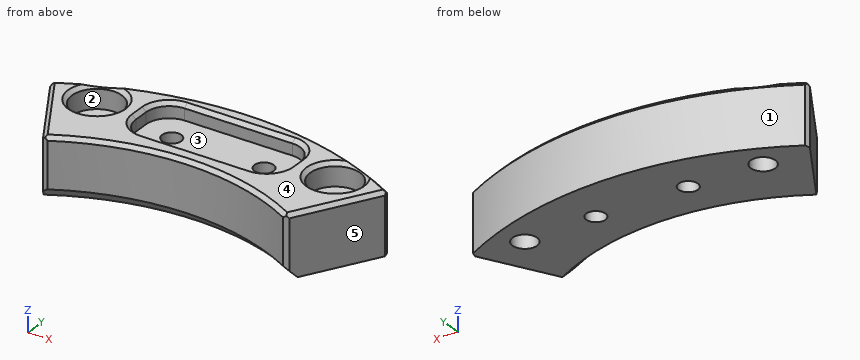
from build123d import *

# Parameters (mm, degrees)
EXTRUDE_1_DEPTH              = 8
CHAMFER_7_SIZE               = 1.5
HOLE_WIZARD_M3_1_D           = 3.2
HOLE_WIZARD_M3_1_CBORE_D     = 6.5
HOLE_WIZARD_M3_1_CBORE_DEPTH = 3
CUT_EXTRUDE_6_DEPTH          = 2
CHAMFER_8_SIZE               = 0.5
CHAMFER_9_SIZE               = 0.5
M3X0_5_1_D                   = 2.5
M3X0_5_1_DEPTH               = 8.5
M3X0_5_1_TIP                 = 0.751075774


with BuildPart() as part:
    # ｽｹｯﾁ3 → ﾎﾞｽ - 押し出し1 (new body)
    with BuildSketch(Plane.XY.offset(-16.5)):
        with BuildLine():
            Line((58.49999999, 38.105482977), (64.74999999, 27.280165429))
            ThreePointArc((64.74999999, 27.280165429), (80.49999999, 31.50036521), (96.24999999, 27.280165429))
            Line((96.24999999, 27.280165429), (102.49999999, 38.105482977))
            ThreePointArc((102.49999999, 38.105482977), (80.49999999, 44.00036521), (58.49999999, 38.105482977))
        make_face()
    extrude(amount=EXTRUDE_1_DEPTH)

    # 面取り7
    chamfer_7_edges = [part.edges().sort_by_distance(p)[0] for p in [
        (80.49999999, 31.50036521, -16.5),
    ]]
    chamfer(chamfer_7_edges, length=CHAMFER_7_SIZE)

    # M3 穴付きねじ用座ぐり穴1 (through all)
    with Locations(Plane.XY.offset(-8.5)):
        with Locations((65.0229264, 37.390950693), (95.977073581, 37.390950693)):
            CounterBoreHole(HOLE_WIZARD_M3_1_D / 2, HOLE_WIZARD_M3_1_CBORE_D / 2, HOLE_WIZARD_M3_1_CBORE_DEPTH)

    # ｽｹｯﾁ17 → ｶｯﾄ - 押し出し6 (cut)
    with BuildSketch(Plane.XY.offset(-8.5)):
        with BuildLine():
            Line((73.49999999, 41.75036521), (87.49999999, 41.75036521))
            ThreePointArc((87.49999999, 41.75036521), (89.621320334, 40.871685554), (90.49999999, 38.75036521))
            Line((90.49999999, 38.75036521), (90.49999999, 36.75036521))
            ThreePointArc((90.49999999, 36.75036521), (89.621320334, 34.629044867), (87.49999999, 33.75036521))
            Line((87.49999999, 33.75036521), (73.49999999, 33.75036521))
            ThreePointArc((73.49999999, 33.75036521), (71.378679647, 34.629044867), (70.49999999, 36.75036521))
            Line((70.49999999, 36.75036521), (70.49999999, 38.75036521))
            ThreePointArc((70.49999999, 38.75036521), (71.378679647, 40.871685554), (73.49999999, 41.75036521))
        make_face()
    extrude(amount=-CUT_EXTRUDE_6_DEPTH, mode=Mode.SUBTRACT)

    # 面取り8
    # the kernel refuses this chamfer: 0.5 mm, written as the material it takes off along each edge
    with BuildSketch(Plane(origin=(80.49999999, 0.00036521, -8.5), x_dir=(-0.5349312949950591, 0.844895561377209, 0), z_dir=(-0.844895561377209, -0.5349312949950591, 0))) as chamfer_8_piece_1:
        Polygon((31.5, CHAMFER_8_SIZE), (31.5 + CHAMFER_8_SIZE, 0), (31.5, 0), align=None)
    revolve(axis=Axis((80.49999999, 0.00036521, -8.5), (0, 0, -1)), revolution_arc=64.678504259, mode=Mode.SUBTRACT)
    with BuildSketch(Plane(origin=(95.607079243, 26.16659403, -8.5), x_dir=(-0.8660254037844379, 0.5000000000000012, 0), z_dir=(0.5000000000000012, 0.866025403784438, 0))) as chamfer_8_piece_2:
        Polygon((CHAMFER_8_SIZE, 0), (0, -CHAMFER_8_SIZE), (0, 0), align=None)
    extrude(amount=15.071682988, mode=Mode.SUBTRACT)
    with BuildSketch(Plane(origin=(80.49999999, 0.00036521, -8.5), x_dir=(0.5250957878127545, 0.8510431326444641, 0), z_dir=(0.8510431326444641, -0.5250957878127545, 0))) as chamfer_8_piece_3:
        Polygon((44 - CHAMFER_8_SIZE, 0), (44, -CHAMFER_8_SIZE), (44, 0), align=None)
    revolve(axis=Axis((80.49999999, 0.00036521, -8.5), (0, 0, 1)), revolution_arc=63.349383731, mode=Mode.SUBTRACT)
    with BuildSketch(Plane(origin=(95.977073581, 37.390950693, -8.5), x_dir=(1, 0, 0), z_dir=(0, -1, 0))) as chamfer_8_piece_4:
        Polygon((3.25 + CHAMFER_8_SIZE, 0), (3.25, -CHAMFER_8_SIZE), (3.25, 0), align=None)
    revolve(axis=Axis((95.977073581, 37.390950693, -8.5), (0, 0, 1)), mode=Mode.SUBTRACT)
    with BuildSketch(Plane(origin=(65.0229264, 37.390950693, -8.5), x_dir=(1, 0, 0), z_dir=(0, -1, 0))) as chamfer_8_piece_5:
        Polygon((3.25 + CHAMFER_8_SIZE, 0), (3.25, -CHAMFER_8_SIZE), (3.25, 0), align=None)
    revolve(axis=Axis((65.0229264, 37.390950693, -8.5), (0, 0, 1)), mode=Mode.SUBTRACT)
    with BuildSketch(Plane(origin=(57.857079243, 39.219054376, -8.5), x_dir=(0, 0, -1), z_dir=(0.5000000000000007, -0.8660254037844384, 0))) as chamfer_8_piece_6:
        Polygon((CHAMFER_8_SIZE, 0), (0, CHAMFER_8_SIZE), (0, 0), align=None)
    extrude(amount=15.071682988, mode=Mode.SUBTRACT)
    with BuildSketch(Plane(origin=(87.49999999, 38.75036521, -8.5), x_dir=(0, 1, 0), z_dir=(-1, 0, 0))) as chamfer_8_piece_7:
        Polygon((3 + CHAMFER_8_SIZE, 0), (3, CHAMFER_8_SIZE), (3, 0), align=None)
    revolve(axis=Axis((87.49999999, 38.75036521, -8.5), (0, 0, -1)), revolution_arc=90, mode=Mode.SUBTRACT)
    with BuildSketch(Plane(origin=(73.49999999, 41.75036521, -8.5), x_dir=(0, 1, 0), z_dir=(1, 0, 0)), Plane(origin=(87.49999999, 33.75036521, -8.5), x_dir=(0, -1, 0), z_dir=(-1, 0, 0))) as chamfer_8_piece_8:
        Polygon((CHAMFER_8_SIZE, 0), (0, -CHAMFER_8_SIZE), (0, 0), align=None)
    extrude(amount=14, mode=Mode.SUBTRACT)
    with BuildSketch(Plane(origin=(73.49999999, 38.75036521, -8.5), x_dir=(-1, 0, 0), z_dir=(0, -1, 0))) as chamfer_8_piece_9:
        Polygon((3 + CHAMFER_8_SIZE, 0), (3, CHAMFER_8_SIZE), (3, 0), align=None)
    revolve(axis=Axis((73.49999999, 38.75036521, -8.5), (0, 0, -1)), revolution_arc=90, mode=Mode.SUBTRACT)
    with BuildSketch(Plane(origin=(70.49999999, 36.75036521, -8.5), x_dir=(-1, 0, 0), z_dir=(0, 1, 0)), Plane(origin=(90.49999999, 38.75036521, -8.5), x_dir=(1, 0, 0), z_dir=(0, -1, 0))) as chamfer_8_piece_10:
        Polygon((CHAMFER_8_SIZE, 0), (0, -CHAMFER_8_SIZE), (0, 0), align=None)
    extrude(amount=2, mode=Mode.SUBTRACT)
    with BuildSketch(Plane(origin=(73.49999999, 36.75036521, -8.5), x_dir=(0, -1, 0), z_dir=(1, 0, 0))) as chamfer_8_piece_11:
        Polygon((3 + CHAMFER_8_SIZE, 0), (3, CHAMFER_8_SIZE), (3, 0), align=None)
    revolve(axis=Axis((73.49999999, 36.75036521, -8.5), (0, 0, -1)), revolution_arc=90, mode=Mode.SUBTRACT)
    with BuildSketch(Plane(origin=(87.49999999, 36.75036521, -8.5), x_dir=(1, 0, 0), z_dir=(0, 1, 0))) as chamfer_8_piece_12:
        Polygon((3 + CHAMFER_8_SIZE, 0), (3, CHAMFER_8_SIZE), (3, 0), align=None)
    revolve(axis=Axis((87.49999999, 36.75036521, -8.5), (0, 0, -1)), revolution_arc=90, mode=Mode.SUBTRACT)

    # 面取り9
    # the kernel refuses this chamfer: 0.5 mm, written as the material it takes off along each edge
    with BuildSketch(Plane(origin=(96.24999999, 27.280165429, -16.296233904), x_dir=(-0.8699980733677616, 0.4930551209919465, 0), z_dir=(0, 0, 1))) as chamfer_9_piece_1:
        with BuildLine():
            Line((0.504048916, 0), (-CHAMFER_9_SIZE * 0.00800077643885, -CHAMFER_9_SIZE * 0.999967993276))
            Line((-CHAMFER_9_SIZE * 0.00800077643885, -CHAMFER_9_SIZE * 0.999967993276), (0, 0))
            ThreePointArc((0, 0), (0.259153689, -0.001007405), (0.504048916, 0))
        make_face()
    extrude(amount=8.592467809, mode=Mode.SUBTRACT)
    with BuildSketch(Plane(origin=(64.74999999, 27.280165429, -16.296233904), x_dir=(-0.499999999999999, 0.8660254037844393, 0), z_dir=(0, 0, 1))) as chamfer_9_piece_2:
        with BuildLine():
            Line((CHAMFER_9_SIZE, 0), (-0.004032783, -0.504032783))
            ThreePointArc((-0.004032783, -0.504032783), (-0.001066058, -0.259153454), (0, 0))
            Line((0, 0), (CHAMFER_9_SIZE, 0))
        make_face()
    extrude(amount=8.592467809, mode=Mode.SUBTRACT)
    with BuildSketch(Plane(origin=(58.49999999, 38.105482977, -17.785841494), x_dir=(0.5000000000000021, -0.8660254037844375, 0), z_dir=(0, 0, 1))) as chamfer_9_piece_3:
        with BuildLine():
            Line((CHAMFER_9_SIZE, 0), (0.002809166, 0.497190834))
            ThreePointArc((0.002809166, 0.497190834), (0.000742578, 0.255629249), (0, 0))
            Line((0, 0), (CHAMFER_9_SIZE, 0))
        make_face()
    extrude(amount=10.071682988, mode=Mode.SUBTRACT)
    with BuildSketch(Plane(origin=(102.49999999, 38.105482977, -17.785841494), x_dir=(-0.8688365739050292, 0.4950989879256175, 0), z_dir=(0, 0, 1))) as chamfer_9_piece_4:
        with BuildLine():
            Line((0.49719877, 0), (CHAMFER_9_SIZE * 0.00564998602096, CHAMFER_9_SIZE * 0.999984038702))
            Line((CHAMFER_9_SIZE * 0.00564998602096, CHAMFER_9_SIZE * 0.999984038702), (0, 0))
            ThreePointArc((0, 0), (0.255629364, -0.000701736), (0.49719877, 0))
        make_face()
    extrude(amount=10.071682988, mode=Mode.SUBTRACT)

    # M3x0.5 ねじ穴1
    with Locations(Plane.XY.offset(-10.5)):
        with Locations((74.49999999, 37.75036521), (86.49999999, 37.75036521)):
            Hole(M3X0_5_1_D / 2, depth=M3X0_5_1_DEPTH)
            with Locations((0, 0, -(M3X0_5_1_DEPTH + M3X0_5_1_TIP / 2))):  # 118° drill point
                Cone(0, M3X0_5_1_D / 2, M3X0_5_1_TIP, mode=Mode.SUBTRACT)


solid = part.part
Geometry: final body of the model. Coordinates: model frame, mm. Face numbers are marked on the shaded views. A direction names the side the tool comes from. Round coordinates to 2 decimals unless told otherwise and drop trailing zeros. Order: outer loops, then holes, each group sorted by start corner. A loop starts at its lowest first (then second) coordinate and runs counter-clockwise, first axis right, second up. Notation, with made-up numbers: (33, 27) -> (41, 27) arc R9 cw to (41, 44) -> close; hole circle Ø2 at (-39, -6). An arc over 180 degrees is marked (long way). Put each result on its own line as item: value. Start each with the question number.
Q1. Pull-direction query (Y, two-part tool) for the marked faces 3, 4 and 5; classes: +Y half, -Y half, draft (parallel to the pull), parting line (faces both ways), or undercut.
Q2. Section B-B on z = -12. Return the cut outline in (x, y).
Q3. Line query: probe 1 along X at (y, z) = (36.5, -10); probe 2 along Z at (x, y) = (80.5, 32); probe 3 along X at (y, z) = (28.5, -13). Output: solid intervals per line, ascending.
Q4. Reachability of the marked faces 1 and 2 from +Z, -Z, +X, -X, +Y, -Y: full face, straight path, thin tool, end or side. Return the list, or none.
Q5. Section A-A on z = -9.75. Return the cut outline in (x, y), and give its area (3 significant figures).
Q6. First-contact query: pin 1 (0.8 mm diameter, centred on x = 78.5, z = -9.5, fed in from +Y); pin 2 (2.5 mm diameter, centred on x = 81, y = 39, fed in from +Z); pin 3 (3 mm diameter, centred on x = 64.5, y = 38, fed in from +Z). Flat tips, straight axial feed; report the tip coordinate or a pass-through.
Ans:
1. face 3: undercut
1. face 4: draft
1. face 5: -Y half
2. outline: (58.75, 37.67) -> (64.5, 27.71) -> (65.19, 27.53) arc R31.5 cw to (95.81, 27.53) -> (96.5, 27.71) -> (102.25, 37.67) -> (102.07, 38.35) arc R44 ccw to (58.93, 38.35) -> close; hole circle Ø3.2 at (65.02, 37.39); hole circle Ø2.5 at (74.5, 37.75); hole circle Ø2.5 at (86.5, 37.75); hole circle Ø3.2 at (95.98, 37.39)
3. probe 1: x = 59.43 to 61.9, 68.15 to 70.51, 90.49 to 92.85, 99.1 to 101.57
3. probe 2: z = -15.5 to -8.5
3. probe 3: x = 64.05 to 67.08, 93.92 to 96.95
4. face 1: +Z, -Z, +Y
4. face 2: +Z
5. outline: (58.75, 37.67) -> (64.5, 27.71) -> (65.19, 27.53) arc R31.5 cw to (95.81, 27.53) -> (96.5, 27.71) -> (102.25, 37.67) -> (102.07, 38.35) arc R44 ccw to (58.93, 38.35) -> close; hole circle Ø6.5 at (65.02, 37.39); hole (70.5, 36.75) arc R3 ccw to (73.5, 33.75) -> (87.5, 33.75) arc R3 ccw to (90.5, 36.75) -> (90.5, 38.75) arc R3 ccw to (87.5, 41.75) -> (73.5, 41.75) arc R3 ccw to (70.5, 38.75) -> close; hole circle Ø6.5 at (95.98, 37.39)
5. area: 275 mm2
6. pin 1: stops at y = 43.97
6. pin 2: stops at z = -10.5
6. pin 3: stops at z = -11.5
